```python
from build123d import *

# Parameters (mm, degrees)
F0_R     = 2.5
F0_R_2   = 2.04
F1_DEPTH = 1
F2_R     = 2.5
F2_R_2   = 2.04
F3_DEPTH = 1


with BuildPart() as f1:
    # F0 (on Top) → F1 (new body)
    with BuildSketch(Plane.XY):
        Circle(F0_R)
        Circle(F0_R_2, mode=Mode.SUBTRACT)
    extrude(amount=F1_DEPTH)

    # F2 (on face) → F3 (join)
    with BuildSketch(Plane(origin=(0, 0, 0), x_dir=(1, 0, 0), z_dir=(0, 0, -1))):
        with BuildLine():
            ThreePointArc((0, -5), (3.5355339059, -3.5355339059), (5, 0))
            ThreePointArc((5, 0), (3.5355339059, 3.5355339059), (0, 5))
            ThreePointArc((0, 5), (-3.5355339059, 3.5355339059), (-5, 0))
            ThreePointArc((-5, 0), (-3.5355339059, -3.5355339059), (0, -5))
        make_face()
        Circle(F2_R, mode=Mode.SUBTRACT)
        with BuildLine():
            Line((5, -5), (5, 0))
            ThreePointArc((5, 0), (3.5355339059, -3.5355339059), (0, -5))
            Line((0, -5), (5, -5))
        make_face()
        with BuildLine():
            ThreePointArc((0, 5), (3.5355339059, 3.5355339059), (5, 0))
            Line((5, 0), (5, 5))
            Line((5, 5), (0, 5))
        make_face()
        with BuildLine():
            ThreePointArc((-5, 0), (-3.5355339059, 3.5355339059), (0, 5))
            Line((0, 5), (-5, 5))
            Line((-5, 5), (-5, 0))
        make_face()
        with BuildLine():
            Line((-5, -5), (0, -5))
            ThreePointArc((0, -5), (-3.5355339059, -3.5355339059), (-5, 0))
            Line((-5, 0), (-5, -5))
        make_face()
        Circle(F2_R)
        Circle(F2_R_2, mode=Mode.SUBTRACT)
    extrude(amount=F3_DEPTH)


solid = f1.part
```
Input: part model. Units: mm. Frame: model coordinates. A direction names the side the tool comes from. Coordinates: 2 decimals unless noted, no trailing zeros. Loops run counter-clockwise (first coordinate to the right, second up) from the corner with the lowest first, then second, coordinate; pieces in that order, holes last. Notation, with made-up numbers: M 7.5,65.5 L 41.5,65.5 A17 ccw 41.5,90.5 Z; hole C 50,-32 d10. An arc over 180 degrees is marked long. Answer in a Markdown table with one row per item.
1. Section C-C, the plane z = -0.85. Output: boundary loops of the cut face in (x, y), then the cut area to 3 significant figures.
Response:
| item | result |
|---|---|
| outline | M -5,-5 L 5,-5 L 5,5 L -5,5 Z; hole C 0,0 d4.08 |
| area | 86.9 mm2 |
2. Section A-A, the plane y = 0. Output: boundary loops of the cut face in (x, z), then the cut area to 3 significant figures.
Response:
| item | result |
|---|---|
| outline | M -5,-1 L -2.04,-1 L -2.04,1 L -2.5,1 L -2.5,0 L -5,0 Z; M 2.04,-1 L 5,-1 L 5,0 L 2.5,0 L 2.5,1 L 2.04,1 Z |
| area | 6.84 mm2 |
3. Material intervals for line 1 (X direction, y = 0, z = -0.1); line 2 (Y direction, x = 0, z = 0.2); line 3 (Z direction, x = -3.5, y = 2.75), sorted ascending.
Response:
| item | result |
|---|---|
| line 1 | x = -5 to -2.04, 2.04 to 5 |
| line 2 | y = -2.5 to -2.04, 2.04 to 2.5 |
| line 3 | z = -1 to 0 |
4. Draft query along Y for faces 3 (the cylindrical face through (-1.62, 1.24, 0.01)), 4 (the flat face through (-5, -0.1, -0.5)), 5 (the cylindrical face through (-0.54, -2.44, 0.49)). Return one class per face: pulls with the +Y half, pulls with the -Y half, needs draft (parallel to the pull), parting line crosses it, or undercut.
Response:
| item | result |
|---|---|
| face 3 | undercut |
| face 4 | needs draft |
| face 5 | parting line crosses it |
5. Section D-D, the plane y = -4. Output: boundary loops of the cut face in (x, z), then the cut area to 3 significant figures.
Response:
| item | result |
|---|---|
| outline | M -5,-1 L 5,-1 L 5,0 L -5,0 Z |
| area | 10.0 mm2 |
6. Reachability of faces 1 (the flat face through (-2, -2, 0)), 2 (the flat face through (0.1, -5, -0.5)) from +Z, -Z, +X, -X, +Y, -Y: full face, straight path, thin tool, end or side. Return the list, or none.
Response:
| item | result |
|---|---|
| face 1 | +Z |
| face 2 | +Z, -Z, +X, -X, -Y |
